```python
from build123d import *

# Parameters (mm, degrees)
SKETCH_1_R      = 3.4
SKETCH_1_R_2    = 2.25
EXTRUDE_1_DEPTH = 4.85
EXTRUDE_START   = 0.5
SKETCH_2_R      = 2.25
SKETCH_2_R_2    = 0.5
EXTRUDE_2_DEPTH = 2
EXTRUDE_START_2 = 1.25
SKETCH_3_R      = 2.25
SKETCH_3_R_2    = 1.15
EXTRUDE_3_DEPTH = 0.9


with BuildPart() as part:
    # 草图1 → 凸台-拉伸1 (new body)
    with BuildSketch(Plane(origin=(0, 0, 0), x_dir=(1, 0, 0), z_dir=(0, 1, 0))):
        with Locations(Location((0, 0, 0), (0, 0, 270))):
            Circle(SKETCH_1_R)
        with Locations(Location((0, 0, 0), (0, 0, 270))):
            Circle(SKETCH_1_R_2, mode=Mode.SUBTRACT)
    extrude(amount=EXTRUDE_1_DEPTH)

    # 草图2 → 凸台-拉伸2 (add)
    with BuildSketch(Plane(origin=(0, 0, 0), x_dir=(1, 0, 0), z_dir=(0, 1, 0)).offset(EXTRUDE_START)):
        with BuildLine():
            Line((1.799999992, 3.407857144), (1.799999992, 6.35))
            ThreePointArc((1.799999992, 6.35), (0, 8.149999992), (-1.799999992, 6.35))
            Line((-1.799999992, 6.35), (-1.799999992, 3.407857144))
            Line((-1.799999992, 3.407857144), (-15.558352909, 2.130295801))
            ThreePointArc((-15.558352909, 2.130295801), (-17.5, 0), (-15.558352909, -2.130295801))
            Line((-15.558352909, -2.130295801), (-1.799999992, -3.407857144))
            Line((-1.799999992, -3.407857144), (-1.799999992, -6.35))
            ThreePointArc((-1.799999992, -6.35), (0, -8.149999992), (1.799999992, -6.35))
            Line((1.799999992, -6.35), (1.799999992, -3.407857144))
            Line((1.799999992, -3.407857144), (15.558352909, -2.130295801))
            ThreePointArc((15.558352909, -2.130295801), (17.5, 0), (15.558352909, 2.130295801))
            Line((15.558352909, 2.130295801), (1.799999992, 3.407857144))
        make_face()
        with Locations(Location((0, 0, 0), (0, 0, 270))):
            Circle(SKETCH_2_R, mode=Mode.SUBTRACT)
        with Locations(Location((0, -6.75, 0), (0, 0, 270))):
            Circle(SKETCH_2_R_2, mode=Mode.SUBTRACT)
        with Locations(Location((0, -4.75, 0), (0, 0, 270))):
            Circle(SKETCH_2_R_2, mode=Mode.SUBTRACT)
        with Locations(Location((15, 0, 0), (0, 0, 270))):
            Circle(SKETCH_2_R_2, mode=Mode.SUBTRACT)
        with Locations(Location((13, 0, 0), (0, 0, 270))):
            Circle(SKETCH_2_R_2, mode=Mode.SUBTRACT)
        with Locations(Location((11, 0, 0), (0, 0, 270))):
            Circle(SKETCH_2_R_2, mode=Mode.SUBTRACT)
        with Locations(Location((9, 0, 0), (0, 0, 270))):
            Circle(SKETCH_2_R_2, mode=Mode.SUBTRACT)
        with Locations(Location((7, 0, 0), (0, 0, 270))):
            Circle(SKETCH_2_R_2, mode=Mode.SUBTRACT)
        with Locations(Location((5, 0, 0), (0, 0, 270))):
            Circle(SKETCH_2_R_2, mode=Mode.SUBTRACT)
        with Locations(Location((0, 6.75, 0), (0, 0, 270))):
            Circle(SKETCH_2_R_2, mode=Mode.SUBTRACT)
        with Locations(Location((0, 4.75, 0), (0, 0, 270))):
            Circle(SKETCH_2_R_2, mode=Mode.SUBTRACT)
        with Locations(Location((-5, 0, 0), (0, 0, 270))):
            Circle(SKETCH_2_R_2, mode=Mode.SUBTRACT)
        with Locations(Location((-7, 0, 0), (0, 0, 270))):
            Circle(SKETCH_2_R_2, mode=Mode.SUBTRACT)
        with Locations(Location((-9, 0, 0), (0, 0, 270))):
            Circle(SKETCH_2_R_2, mode=Mode.SUBTRACT)
        with Locations(Location((-11, 0, 0), (0, 0, 270))):
            Circle(SKETCH_2_R_2, mode=Mode.SUBTRACT)
        with Locations(Location((-13, 0, 0), (0, 0, 270))):
            Circle(SKETCH_2_R_2, mode=Mode.SUBTRACT)
        with Locations(Location((-15, 0, 0), (0, 0, 270))):
            Circle(SKETCH_2_R_2, mode=Mode.SUBTRACT)
    extrude(amount=EXTRUDE_2_DEPTH)

    # 草图3 → 凸台-拉伸3 (add)
    with BuildSketch(Plane(origin=(0, 0, 0), x_dir=(1, 0, 0), z_dir=(0, 1, 0)).offset(EXTRUDE_START_2)):
        with Locations(Location((0, 0, 0), (0, 0, 270))):
            Circle(SKETCH_3_R)
        with Locations(Location((0, 0, 0), (0, 0, 270))):
            Circle(SKETCH_3_R_2, mode=Mode.SUBTRACT)
    extrude(amount=EXTRUDE_3_DEPTH)


solid = part.part
```
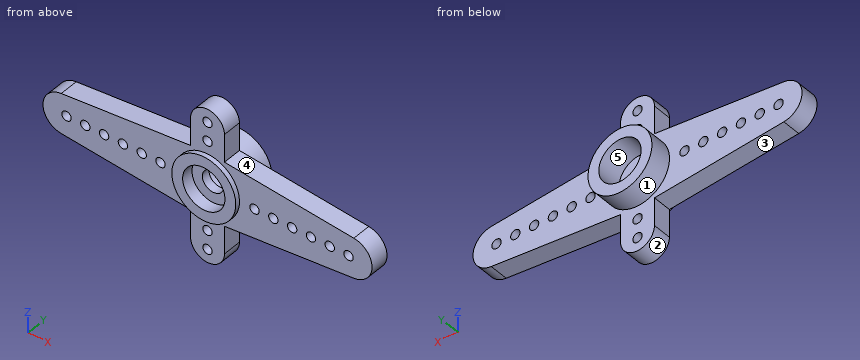
Geometry check sheet. Reference: the model listing, model coordinates, mm. Face numbers are marked on the shaded views. A direction names the side the tool comes from. Coordinates: 2 decimals unless noted, no trailing zeros. Write each loop counter-clockwise with the first axis right and the second up, starting at its lowest first coordinate (ties: lowest second). Pieces come first, ordered by that corner, then holes. Notation, with made-up numbers: M 39,-3.75 L 59,-3.75 A10 cw 59,10.25 Z; hole C -37,73.25 d4. An arc over 180 degrees is marked long. One line per item, written item: value. Start each with the question number.
(1) Tool access check on the marked faces 1 and 2. Record the directions out of +Z, -Z, +X, -X, +Y, -Y that give a thin tool (end or side, any length) a straight path to the whole face; none if there is none.
(2) Release check for a two-part mould opening along Z. For the marked faces 3, 4 and 5 record: released by +Z, released by -Z, zero draft, split by the parting line, or undercut.
(3) Sectioned sample at B-B, the plane x = -13. Enter the section's corners in (y, z), and give its area (3 significant figures).
(4) Sectioned sample at C-C, the plane x = 0. State how many separate pieces and enclosed holes the cut face has, and give its area (3 significant figures).
(5) Scan lines: line 1 along X through (y, z) = (3.5, 0); line 2 along Y through (x, z) = (13, 2); line 3 along X through (y, z) = (1.2, 5.5). Record each from-to range of solid material in increasing order. Write a range as [from, to].
(6) Sectioned sample at D-D, the plane y = 3.7. Enter the section's corners in (x, z), and give its area (3 significant figures).
(7) Sectioned sample at A-A, the plane z = -4.75. Enter the section's corners in (x, y).
(8) Depth check by flat-ended pin: pin 1 (2 mm diameter, centred on x = -3.5, y = 2, fed in from +Z); pin 2 (1.5 mm diameter, centred on x = 1, y = 1.5, fed in from -Z); pin 3 (5 mm diameter, centred on x = 6.5, z = -0.5, fed in from +Y). Enter the tip coordinate at first touch or a pass-through.
Filled sheet:
1. face 1: +Y
1. face 2: -Z, +Y, -Y
2. face 3: released by -Z
2. face 4: released by +Z
2. face 5: undercut
3. outline: M 0.5,-2.37 L 2.5,-2.37 L 2.5,-0.5 L 0.5,-0.5 Z; M 0.5,0.5 L 2.5,0.5 L 2.5,2.37 L 0.5,2.37 Z
3. area: 7.47 mm²
4. separate pieces: 6
4. enclosed holes: 0
4. area: 24.1 mm²
5. line 1: [-3.4, -2.25], [2.25, 3.4]
5. line 2: [0.5, 2.5]
5. line 3: [-1.8, 1.8]
6. outline: C 0,0 d6.8; hole C 0,0 d4.5
6. area: 20.4 mm²
7. outline: M -1.8,0.5 L -0.5,0.5 L -0.5,2.5 L -1.8,2.5 Z; M 0.5,0.5 L 1.8,0.5 L 1.8,2.5 L 0.5,2.5 Z
8. pin 1: z = 3.34
8. pin 2: z = -8.13
8. pin 3: y = 2.5
